Could you check a few things on this model? Use its own coordinates, in mm. A direction names the side the tool comes from. Round coordinates to 2 decimals unless told otherwise and drop trailing zeros. Order: outer loops, then holes, each group sorted by start corner. A loop starts at its lowest first (then second) coordinate and runs counter-clockwise, first axis right, second up. Notation, with made-up numbers: (83, 54) -> (113, 54) arc R20 ccw to (113, 87) -> close; hole circle Ø11 at (83.5, 51.5). An arc over 180 degrees is marked (long way). Put each result on its own line as item: value. Start each with the question number.
from build123d import *

# Parameters (mm, degrees)
SKETCH_1_W             = 45
SKETCH_1_H             = 10
EXTRUDE_1_DEPTH        = 2
SKETCH_2_W             = 45
SKETCH_2_H             = 23
EXTRUDE_2_DEPTH        = 2
SKETCH_4_W             = 45
SKETCH_4_H             = 2
EXTRUDE_3_DEPTH        = 10
PATTERN_LINEAR_1_COUNT = 3
PATTERN_LINEAR_1_PITCH = 10
HOLE_WIZARD_M3_2_DEPTH = 2
SKETCH_9_W             = 8
SKETCH_9_H             = 2
CUT_EXTRUDE_1_DEPTH    = 30.904013109
FILLET_1_R             = 6
FILLET_3_R             = 1
CUT_EXTRUDE_2_REACH    = 31.904
SKETCH_11_W            = 8
SKETCH_11_H            = 11
FILLET_5_R             = 1


# Read off the part's stored shape, not the designer's step: M3 间隙槽口2
with BuildPart() as part:
    # 草图1 → 凸台-拉伸1 (new body)
    with BuildSketch(Plane.XY):
        Rectangle(SKETCH_1_W, SKETCH_1_H)
    extrude(amount=EXTRUDE_1_DEPTH)

    # 草图2 → 凸台-拉伸2 (add)
    with BuildSketch(Plane.XY):
        with Locations((0, -6.5)):
            Rectangle(SKETCH_2_W, SKETCH_2_H)
    extrude(amount=EXTRUDE_2_DEPTH)

    # 草图4 → 凸台-拉伸3 (add)
    with BuildSketch(Plane.XY):
        with Locations((0, -17)):
            Rectangle(SKETCH_4_W, SKETCH_4_H)
    extrude(amount=EXTRUDE_3_DEPTH)

    # 草图6 → M3 间隙孔1 (revolve, cut)
    with BuildSketch(Plane(origin=(-10, -16, 6), x_dir=(0, 0, 1), z_dir=(1, 0, 0))):
        Polygon((0, 0), (0, 9.521463052), (1.7, 8.5), (1.7, 0), align=None)
    hole_wizard_m3_1 = revolve(axis=Axis((-10, -9.65, 6), (0, -1, 0)), mode=Mode.SUBTRACT)

    # 阵列(线性)1: M3 间隙孔1 ×3
    with Locations(*[(i * PATTERN_LINEAR_1_PITCH, 0, 0) for i in range(1, PATTERN_LINEAR_1_COUNT)]):
        add(hole_wizard_m3_1, mode=Mode.SUBTRACT)

    # M3 间隙槽口2 outline → M3 间隙槽口2 (cut)
    with BuildSketch(Plane.XY):
        with BuildLine():
            ThreePointArc((20.2, 1.3), (18.5, 3), (16.8, 1.3))
            Line((16.8, 1.3), (16.8, -3.3))
            ThreePointArc((16.8, -3.3), (18.5, -5), (20.2, -3.3))
            Line((20.2, -3.3), (20.2, 1.3))
        make_face()
        with BuildLine():
            ThreePointArc((-16.8, 1.3), (-18.5, 3), (-20.2, 1.3))
            Line((-20.2, 1.3), (-20.2, -3.3))
            ThreePointArc((-20.2, -3.3), (-18.5, -5), (-16.8, -3.3))
            Line((-16.8, -3.3), (-16.8, 1.3))
        make_face()
    extrude(amount=HOLE_WIZARD_M3_2_DEPTH, mode=Mode.SUBTRACT)

    # 草图9 → 切除-拉伸1 (cut, through all)
    with BuildSketch(Plane.XY.offset(2)):
        with Locations((-18.5, -17)):
            Rectangle(SKETCH_9_W, SKETCH_9_H)
        with Locations((18.5, -17)):
            Rectangle(SKETCH_9_W, SKETCH_9_H)
    extrude(amount=CUT_EXTRUDE_1_DEPTH, mode=Mode.SUBTRACT)

    # 圆角1
    fillet_1_edges = [part.edges().sort_by_distance(p)[0] for p in [
        (-14.5, -17, 10),
        (14.5, -17, 10),
    ]]
    fillet(fillet_1_edges, radius=FILLET_1_R)

    # 圆角3
    fillet_3_edges = [part.edges().sort_by_distance(p)[0] for p in [
        (0, -16, 2),
    ]]
    fillet(fillet_3_edges, radius=FILLET_3_R)

    # 草图11 → 切除-拉伸2 (cut, up to next)
    with BuildSketch(Plane.XY.offset(2), mode=Mode.PRIVATE) as cut_extrude_2_sk1:
        with Locations((-18.5, -12.5)):
            Rectangle(SKETCH_11_W, SKETCH_11_H)
    cut_extrude_2_tool1 = extrude(cut_extrude_2_sk1.sketch, amount=-CUT_EXTRUDE_2_REACH, mode=Mode.PRIVATE) & part.part
    cut_extrude_2 = cut_extrude_2_tool1.solids().sort_by_distance((-18.5, -12.5, 2))[0]
    add(cut_extrude_2, mode=Mode.SUBTRACT)

    # 镜向1: 切除-拉伸2 across plane
    add(cut_extrude_2.mirror(Plane(origin=(0, 0, 0), x_dir=(0, 0, 1), z_dir=(1, 0, 0))), mode=Mode.SUBTRACT)

    # 圆角5
    fillet_5_edges = [part.edges().sort_by_distance(p)[0] for p in [
        (-22.5, -7, 1),
        (-14.5, -7, 1),
        (22.5, -7, 1),
        (14.5, -7, 1),
        (-22.5, 5, 1),
        (22.5, 5, 1),
    ]]
    fillet(fillet_5_edges, radius=FILLET_5_R)


solid = part.part
1. For pin 1 Ø1.6 at (x, z) = (18.5, 1) entering from -Y; pin 2 Ø4.5 at (y, z) = (-13, 2.5) entering from -X; pin 3 Ø1 at (x, y) = (14, 2) entering from +Z, each with a flat end and sliding along its axis, tell me the tip position at first contact or that it passes through.
2. If we section it at B-B, the plane y = 0: Please give me the cut outline in (x, z).
3. If we section it at D-D, the plane y = -11.25: Please give me the cut outline in (x, z), then the cut area to 3 significant figures.
4. If we section it at A-A, the plane x = 18.5: Please give me the cut outline in (y, z), then the cut area to 3 significant figures.
5. Thinking about a two-plate mould opening in Z: for faces 1 (the face through (18.5, 3, 1)), 2 (the face through (-8.34, -16.99, 5.63)), 3 (the face through (12.789, -17.014, 8.196)), which applies, +Z half, -Z half, draft (parallel to the pull), parting line (faces both ways), or undercut?
6. If we section it at C-C, the plane x = -2.5: Please give me the cut outline in (y, z), then the cut area to 3 significant figures.
7. Which directions (+Z, -Z, +X, -X, +Y, -Y) give clear straight access to the entire face, cutting with the end or side of a thin tool? Please do faces 4 (the face through (-14.5, -14.2, 1.5)), 5 (the face through (0, -16, 8)), 6 (the face through (16.8, -1, 1)), 7 (the face through (19, -7, 1)).
8. I need wall thicknesses on L1, parallel to X at y = -16.65, z = 6; L2, parallel to Z at x = 0, y = -17.55; L3, parallel to Z at x = 11.5, y = -8.75. Which ranges of each line are inside material? Lowest first, please.
Results below:
1. pin 1: y = -7
1. pin 2: x = -14.5
1. pin 3: z = 2
2. outline: (-22.5, 0) -> (-20.2, 0) -> (-20.2, 2) -> (-22.5, 2) -> close; (-16.8, 0) -> (16.8, 0) -> (16.8, 2) -> (-16.8, 2) -> close; (20.2, 0) -> (22.5, 0) -> (22.5, 2) -> (20.2, 2) -> close
3. outline: (-14.5, 0) -> (14.5, 0) -> (14.5, 2) -> (-14.5, 2) -> close
3. area: 58.0 mm2
4. outline: (-7, 0) -> (-5, 0) -> (-5, 2) -> (-7, 2) -> close; (3, 0) -> (5, 0) -> (5, 2) -> (3, 2) -> close
4. area: 8.00 mm2
5. face 1: draft
5. face 2: undercut
5. face 3: +Z half
6. outline: (-18, 0) -> (5, 0) -> (5, 2) -> (-15, 2) arc R1 cw to (-16, 3) -> (-16, 10) -> (-18, 10) -> close
6. area: 62.2 mm2
7. face 4: +Z, -Z, -X, -Y
7. face 5: +Z, +X, -X, +Y
7. face 6: +Z, -Z
7. face 7: +Z, -Z, +X, -Y
8. L1: -14.16 to -11.7, -8.3 to -1.7, 1.7 to 8.3, 11.7 to 14.16
8. L2: 0 to 4.3, 7.7 to 10
8. L3: 0 to 2
